```python
from build123d import *

# Parameters (mm, degrees)
SKETCH1_W         = 87
SKETCH1_H         = 50.982
BASE_YELLOW_DEPTH = 22
SKETCH2_R         = 11
COUNTERBOR_DEPTH  = 4
SKETCH2_5_R       = 8
COUNTERBOR2_DEPTH = 23
SKETCH5_W         = 40
SKETCH5_H         = 38
BASE_RED_DEPTH    = 30
SKETCH7_R         = 15
SKETCH7_W         = 40
SKETCH7_H         = 20
BASE_PURPLE_DEPTH = 20
BASE_TURKIZ_DEPTH = 88


with BuildPart() as part:
    # Sketch1 → base-yellow (new body)
    with BuildSketch(Plane.XY):
        Rectangle(SKETCH1_W, SKETCH1_H)
    extrude(amount=-BASE_YELLOW_DEPTH)

    # Sketch2 → counterbor (cut)
    with BuildSketch(Plane.XY):
        with Locations((-26.5, 0)):
            Circle(SKETCH2_R)
    extrude(amount=-COUNTERBOR_DEPTH, mode=Mode.SUBTRACT)

    # Sketch2_5 → counterbor2 (cut, through all)
    with BuildSketch(Plane.XY):
        with Locations((-26.5, 0)):
            Circle(SKETCH2_5_R)
    extrude(amount=-COUNTERBOR2_DEPTH, mode=Mode.SUBTRACT)

    # Sketch5 → base-red (add)
    with BuildSketch(Plane.XY):
        with Locations((10.5, 0)):
            Rectangle(SKETCH5_W, SKETCH5_H)
    extrude(amount=BASE_RED_DEPTH)

    # Sketch7 → base-purple (cut)
    with BuildSketch(Plane.XY.offset(30)):
        with Locations((10.5, 0)):
            Circle(SKETCH7_R)
        with Locations((10.5, 0)):
            Rectangle(SKETCH7_W, SKETCH7_H)
    extrude(amount=-BASE_PURPLE_DEPTH, mode=Mode.SUBTRACT)

    # Sketch8 → base-turkiz (cut, through all)
    with BuildSketch(Plane.ZY.offset(43.5)):
        Polygon((-10, 10), (-10, -10), (-13, -10), (-13, -17.696152423), (-22, -12.5), (-22, 12.5), (-13, 17.696152423), (-13, 10), align=None)
    extrude(amount=-BASE_TURKIZ_DEPTH, mode=Mode.SUBTRACT)


solid = part.part
```
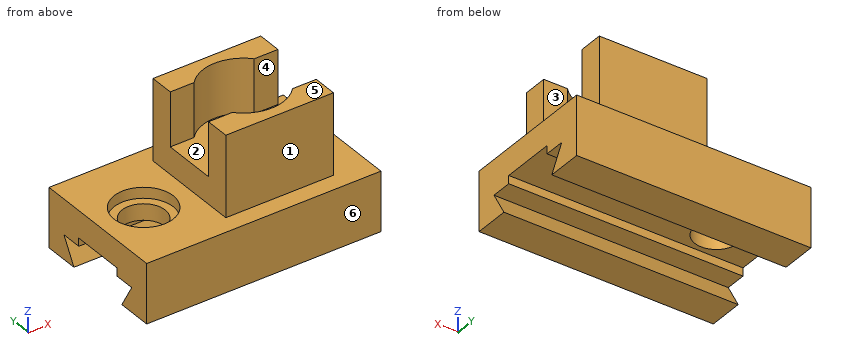
Input: part model. Units: mm. Frame: model coordinates. Face numbers are marked on the shaded views. A direction names the side the tool comes from. Coordinates: 2 decimals unless noted, no trailing zeros. Write each loop counter-clockwise with the first axis right and the second up, starting at its lowest first coordinate (ties: lowest second). Pieces come first, ordered by that corner, then holes.
1) Mould query, pull axis Y, two halves, no side actions, for the marked faces 4, 5 and 6. Classes: pulls with the +Y half, pulls with the -Y half, needs draft (parallel to the pull), parting line crosses it, or undercut.
2) Section A-A on z = 19. Output: boundary loops of the cut face in (x, y).
3) Section D-D on z = -8. Output: boundary loops of the cut face in (x, y), and give its area (3 significant figures).
4) Pin query (flat end, axial travel): pin 1 Ø15 at (x, z) = (2.5, 12.5) entering from -Y; pin 2 Ø4.5 at (x, z) = (26.5, 20.5) entering from +Y; pin 3 Ø10 at (x, y) = (-23.5, -5) entering from +Z. Return the tip coordinate at first contact, or that it passes through.
5) Set-up query: the marked faces 1, 2 and 3. Return all of +Z, -Z, +X, -X, +Y, -Y with unobstructed straight access to the full face (end or side cutting, diameter ignored); none if empty.
6) Section C-C on y = 0. Output: boundary loops of the cut face in (x, z).
7) Section B-B on x = -26.5. Output: boundary loops of the cut face in (y, z), and give its area (3 significant figures).
8) Material intervals for line 1 along Y through (x, z) = (-3.5, -12); line 2 along Y through (x, z) = (-7, 24.5); line 3 along Z through (x, y) = (-35, 6), sorted ascending.
Check result:
1. face 4: undercut
1. face 5: needs draft
1. face 6: pulls with the -Y half
2. outline: (-9.5, -19) - (30.5, -19) - (30.5, -10) - (21.68, -10) arc R15 cw to (-0.68, -10) - (-9.5, -10) - close; (-9.5, 10) - (-0.68, 10) arc R15 cw to (21.68, 10) - (30.5, 10) - (30.5, 19) - (-9.5, 19) - close
3. outline: (-43.5, -25.49) - (43.5, -25.49) - (43.5, 25.49) - (-43.5, 25.49) - close; hole circle Ø16 at (-26.5, 0)
3. area: 4,230 mm2
4. pin 1: stops at y = -19
4. pin 2: stops at y = 19
4. pin 3: stops at z = -4
5. face 1: +Z, +X, -X, -Y
5. face 2: +Z
5. face 3: +Z, +X, -X
6. outline: (-43.5, -10) - (-34.5, -10) - (-34.5, -4) - (-37.5, -4) - (-37.5, 0) - (-43.5, 0) - close; (-18.5, -10) - (43.5, -10) - (43.5, 0) - (30.5, 0) - (30.5, 10) - (-9.5, 10) - (-9.5, 0) - (-15.5, 0) - (-15.5, -4) - (-18.5, -4) - close
7. outline: (-25.49, -22) - (-12.5, -22) - (-17.7, -13) - (-10, -13) - (-10, -10) - (-8, -10) - (-8, -4) - (-11, -4) - (-11, 0) - (-25.49, 0) - close; (8, -10) - (10, -10) - (10, -13) - (17.7, -13) - (12.5, -22) - (25.49, -22) - (25.49, 0) - (11, 0) - (11, -4) - (8, -4) - close
7. area: 606 mm2
8. line 1: y = -25.49 to -10, 10 to 25.49
8. line 2: y = -19 to -10, 10 to 19
8. line 3: z = -10 to -4
